from build123d import *

# Parameters (mm, degrees)
SKETCH1_R           = 2.55
SKETCH1_R_2         = 3.4
BOSS_EXTRUDE1_DEPTH = 205


with BuildPart() as part:
    # Sketch1 → Boss-Extrude1 (new body)
    with BuildSketch(Plane.XY):
        with BuildLine():
            Line((13, 4), (15, 4))
            Line((15, 4), (15, 13))
            ThreePointArc((15, 13), (14.414213562, 14.414213562), (13, 15))
            Line((13, 15), (4, 15))
            Line((4, 15), (4, 13))
            Line((4, 13), (8.25, 13))
            Line((8.25, 13), (8.25, 9.664213562))
            Line((8.25, 9.664213562), (4.585786438, 6))
            Line((4.585786438, 6), (-4.585786438, 6))
            Line((-4.585786438, 6), (-8.25, 9.664213562))
            Line((-8.25, 9.664213562), (-8.25, 13))
            Line((-8.25, 13), (-4, 13))
            Line((-4, 13), (-4, 15))
            Line((-4, 15), (-13, 15))
            ThreePointArc((-13, 15), (-14.414213562, 14.414213562), (-15, 13))
            Line((-15, 13), (-15, 4))
            Line((-15, 4), (-13, 4))
            Line((-13, 4), (-13, 8.25))
            Line((-13, 8.25), (-9.664213562, 8.25))
            Line((-9.664213562, 8.25), (-6, 4.585786438))
            Line((-6, 4.585786438), (-6, -4.585786438))
            Line((-6, -4.585786438), (-9.664213562, -8.25))
            Line((-9.664213562, -8.25), (-13, -8.25))
            Line((-13, -8.25), (-13, -4))
            Line((-13, -4), (-15, -4))
            Line((-15, -4), (-15, -13))
            ThreePointArc((-15, -13), (-14.414213562, -14.414213562), (-13, -15))
            Line((-13, -15), (-4, -15))
            Line((-4, -15), (-4, -13))
            Line((-4, -13), (-8.25, -13))
            Line((-8.25, -13), (-8.25, -9.664213562))
            Line((-8.25, -9.664213562), (-4.585786438, -6))
            Line((-4.585786438, -6), (4.585786438, -6))
            Line((4.585786438, -6), (8.25, -9.664213562))
            Line((8.25, -9.664213562), (8.25, -13))
            Line((8.25, -13), (4, -13))
            Line((4, -13), (4, -15))
            Line((4, -15), (13, -15))
            ThreePointArc((13, -15), (14.414213562, -14.414213562), (15, -13))
            Line((15, -13), (15, -4))
            Line((15, -4), (13, -4))
            Line((13, -4), (13, -8.25))
            Line((13, -8.25), (9.664213562, -8.25))
            Line((9.664213562, -8.25), (6, -4.585786438))
            Line((6, -4.585786438), (6, 4.585786438))
            Line((6, 4.585786438), (9.664213562, 8.25))
            Line((9.664213562, 8.25), (13, 8.25))
            Line((13, 8.25), (13, 4))
        make_face()
        with Locations(Location((-11.6, 11.6, 0), (0, 0, 180))):  # turned: the seam where the file's is
            Circle(SKETCH1_R, mode=Mode.SUBTRACT)
        with Locations(Location((11.6, -11.6, 0), (0, 0, 180))):  # turned: the seam where the file's is
            Circle(SKETCH1_R, mode=Mode.SUBTRACT)
        with Locations(Location((-11.6, -11.6, 0), (0, 0, 180))):  # turned: the seam where the file's is
            Circle(SKETCH1_R, mode=Mode.SUBTRACT)
        with Locations(Location((11.6, 11.6, 0), (0, 0, 180))):  # turned: the seam where the file's is
            Circle(SKETCH1_R, mode=Mode.SUBTRACT)
        with Locations(Location((0, 0, 0), (0, 0, 180))):  # turned: the seam where the file's is
            Circle(SKETCH1_R_2, mode=Mode.SUBTRACT)
    extrude(amount=BOSS_EXTRUDE1_DEPTH)


solid = part.part
Verification items for the finished model (mm, model axes). A direction names the side the tool comes from. Give positions to 0.01 mm unless a question says otherwise; leave off trailing zeros. Write each loop counter-clockwise with the first axis right and the second up, starting at its lowest first coordinate (ties: lowest second). Pieces come first, ordered by that corner, then holes. Notation, with made-up numbers: M 63.5,-35.5 L 68.5,-35.5 A20 ccw 68.5,-25.5 Z; hole C 52.5,47.5 d9. An arc over 180 degrees is marked long. Write item = value, one per line.
(1) Sectioned sample at A-A (x = 0). Record the cut outline in (y, z), then the cut area to 3 significant figures.
Found:
outline = M -6,0 L -3.4,0 L -3.4,205 L -6,205 Z; M 3.4,0 L 6,0 L 6,205 L 3.4,205 Z
area = 1,070 mm2
(2) Sectioned sample at C-C (z = 67). Give the number of separate pieces and of enclosed holes in the cut face, then the cut area to 3 significant figures.
Found:
separate_pieces = 1
enclosed_holes = 5
area = 306 mm2
(3) Material ranges on line 1 (X direction, y = -12, z = 131); line 2 (Y direction, x = 11.6, z = 106.5); line 3 (X direction, y = -9.5, z = 179), recorded low to high.
Found:
line_1 = -15 to -14.12, -9.08 to -8.25, 8.25 to 9.08, 14.12 to 15
line_2 = -15 to -14.15, -9.05 to -8.25, 8.25 to 9.05, 14.15 to 15
line_3 = -15 to -13.05, -10.15 to -8.09, 8.09 to 10.15, 13.05 to 15
(4) Draft check along Y on faces 3 (the face through (9.244, 12.577, 101.065)), 4 (the face through (-1.2, 3.4, 205)). Enter one of: released by +Y, released by -Y, zero draft, split by the parting line, or undercut.
Found:
face_3 = undercut
face_4 = zero draft
(5) Access from +Z, -Z, +X, -X, +Y, -Y to the whole of each face (thin tool, end or side, straight path). Record for faces 1 (the face through (-6, -13, 101)), 2 (the face through (15, 8, 101)).
Found:
face_1 = +Z, -Z
face_2 = +Z, -Z, +X, +Y, -Y
(6) Go/stop test with flat-tipped pins: pin 1 Ø0.6 at (x, z) = (-14.5, 153.5) entering from +Y; pin 2 Ø3 at (x, z) = (-1.5, 95.5) entering from +Y; pin 3 Ø3 at (y, z) = (-1.5, 70) entering from +X. Record where each tip stops, or that it passes through.
Found:
pin_1 = 14.6
pin_2 = 6
pin_3 = 6
